```python
from build123d import *

# Parameters (mm, degrees)
SKETCH1_W           = 500
SKETCH1_H           = 150
SKETCH1_R           = 9.3
SKETCH1_R_2         = 3
SKETCH1_R_3         = 4
BOSS_EXTRUDE1_DEPTH = 6.35
CUT_EXTRUDE1_DEPTH  = 7
SKETCH4_R           = 9.3
CUT_EXTRUDE2_DEPTH  = 10
FILLET1_R           = 2
CUT_EXTRUDE4_DEPTH  = 10
SKETCH6_R           = 1.75
SKETCH6_R_2         = 3
CUT_EXTRUDE5_DEPTH  = 10


with BuildPart() as part:
    # Sketch1 → Boss-Extrude1 (new body)
    with BuildSketch(Plane.XY):
        with Locations((200, 0)):
            Rectangle(SKETCH1_W, SKETCH1_H)
        Circle(SKETCH1_R, mode=Mode.SUBTRACT)
        with BuildLine():
            ThreePointArc((303.793920425, 21.250000148), (340.59999997, 42.5), (377.406079545, 21.250000201))
            ThreePointArc((377.406079545, 21.250000201), (375.758965412, 15.102885723), (369.61185099, 16.750000063))
            ThreePointArc((369.61185099, 16.750000063), (340.600001147, 33.5), (311.588150157, 16.750002051))
            ThreePointArc((311.588150157, 16.750002051), (305.441035607, 15.102885134), (303.793920425, 21.250000148))
        make_face(mode=Mode.SUBTRACT)
        with Locations((377.1687, -9.7841)):
            Circle(SKETCH1_R_2, mode=Mode.SUBTRACT)
        with Locations((340.6, 0)):
            Circle(SKETCH1_R_3, mode=Mode.SUBTRACT)
    extrude(amount=BOSS_EXTRUDE1_DEPTH)

    # Sketch3 → Cut-Extrude1 (cut)
    with BuildSketch(Plane.XY.offset(6.35)):
        with BuildLine():
            Line((36.827355724, 55), (-50, 55))
            Line((-50, 55), (-50, -75))
            Line((-50, -75), (450, -75))
            Line((450, -75), (450, 55))
            Line((450, 55), (340.6, 55))
            ThreePointArc((340.6, 55), (379.490872965, 38.890872965), (395.6, 0))
            ThreePointArc((395.6, 0), (394.766919757, -9.536498518), (392.292916219, -18.7841))
            ThreePointArc((392.292916219, -18.7841), (329.589221669, -53.886573101), (285.681879129, 3))
            Line((285.681879129, 3), (30.896152423, 3))
            Line((30.896152423, 3), (21.172644276, 3))
            Line((21.172644276, 3), (9.086322138, -9.086322138))
            ThreePointArc((9.086322138, -9.086322138), (-9.086322138, -9.086322138), (-9.086322138, 9.086322138))
            Line((-9.086322138, 9.086322138), (36.827355724, 55))
        make_face()
        with BuildLine():
            Line((328.4653389, 3), (285.681879129, 3))
            ThreePointArc((285.681879129, 3), (329.589221669, -53.886573101), (392.292916219, -18.7841))
            Line((392.292916219, -18.7841), (371.532319214, -18.7841))
            Line((371.532319214, -18.7841), (351.002913897, -6.930323401))
            ThreePointArc((351.002913897, -6.930323401), (335.559903988, -11.438856245), (328.4653389, 3))
        make_face()
        Polygon((-50, 75), (-50, 55), (36.827355724, 55), (340.6, 55), (450, 55), (450, 75), align=None)
    extrude(amount=-CUT_EXTRUDE1_DEPTH, mode=Mode.SUBTRACT)

    # Sketch4 → Cut-Extrude2 (cut)
    with BuildSketch(Plane.XY.offset(6.35)):
        with BuildLine():
            Line((23.112698372, 8), (6.470027048, 24.642671324))
            Line((6.470027048, 24.642671324), (-9.086322138, 9.086322138))
            ThreePointArc((-9.086322138, 9.086322138), (4.917482106, 11.871851993), (12.85, 0))
            ThreePointArc((12.85, 0), (11.871851993, -4.917482106), (9.086322138, -9.086322138))
            Line((9.086322138, -9.086322138), (21.172644276, 3))
            Line((21.172644276, 3), (41, 3))
            Line((41, 3), (41, 8))
            Line((41, 8), (23.112698372, 8))
        make_face()
        with BuildLine():
            ThreePointArc((12.85, 0), (4.917482106, 11.871851993), (-9.086322138, 9.086322138))
            ThreePointArc((-9.086322138, 9.086322138), (-9.086322138, -9.086322138), (9.086322138, -9.086322138))
            ThreePointArc((9.086322138, -9.086322138), (11.871851993, -4.917482106), (12.85, 0))
        make_face()
        Circle(SKETCH4_R, mode=Mode.SUBTRACT)
        Polygon((36.827355724, 55), (30.827355724, 49), (50.827355724, 49), (50.827355724, 55), align=None)
    extrude(amount=-CUT_EXTRUDE2_DEPTH, mode=Mode.SUBTRACT)

    # Fillet1
    fillet1_edges = [part.edges().sort_by_distance(p)[0] for p in [
        (328.4653389, 3, 3.175),
        (351.002913897, -6.930323401, 3.175),
        (392.292916219, -18.7841, 3.175),
    ]]
    fillet(fillet1_edges, radius=FILLET1_R)

    # Sketch5 → Cut-Extrude4 (cut)
    with BuildSketch(Plane.XY.offset(6.35)):
        with BuildLine():
            ThreePointArc((328.129761947, 0.862068966), (332.07139701, 9.138540969), (340.6, 12.5))
            Line((340.6, 12.5), (394.160713214, 12.5))
            ThreePointArc((394.160713214, 12.5), (374.786985828, 43.084219849), (340.6, 55))
            Line((340.6, 55), (50.827355724, 55))
            Line((50.827355724, 55), (50.827355724, 49))
            Line((50.827355724, 49), (30.827355724, 49))
            Line((30.827355724, 49), (6.470027048, 24.642671324))
            Line((6.470027048, 24.642671324), (23.112698372, 8))
            Line((23.112698372, 8), (41, 8))
            Line((41, 8), (41, 3))
            Line((41, 3), (326.134523859, 3))
            ThreePointArc((326.134523859, 3), (327.596690413, 2.364576478), (328.129761947, 0.862068966))
        make_face()
        with BuildLine():
            ThreePointArc((311.588150157, 16.750002051), (305.441035607, 15.102885134), (303.793920425, 21.250000148))
            ThreePointArc((303.793920425, 21.250000148), (340.59999997, 42.5), (377.406079545, 21.250000201))
            ThreePointArc((377.406079545, 21.250000201), (375.758965412, 15.102885723), (369.61185099, 16.750000063))
            ThreePointArc((369.61185099, 16.750000063), (340.600001147, 33.5), (311.588150157, 16.750002051))
        make_face(mode=Mode.SUBTRACT)
    extrude(amount=-CUT_EXTRUDE4_DEPTH, mode=Mode.SUBTRACT)


with BuildPart() as cut_extrude4_kept_piece:
    # of the separate pieces the step leaves, the one the design keeps (cut_extrude4_pieces_kept)
    add(part.part.solids().sort_by_distance((340.6, 12.5, 0))[0])

    # Sketch6 → Cut-Extrude5 (cut)
    with BuildSketch(Plane.XY.offset(6.35)):
        with Locations((350.6, 7.5)):
            Circle(SKETCH6_R)
        with Locations((387.1687, 0)):
            Circle(SKETCH6_R)
        with Locations((377.1687, -9.7841)):
            Circle(SKETCH6_R_2)
        with Locations((365.870678247, -10.944141097)):
            Circle(SKETCH6_R)
    extrude(amount=-CUT_EXTRUDE5_DEPTH, mode=Mode.SUBTRACT)


solid = cut_extrude4_kept_piece.part
```
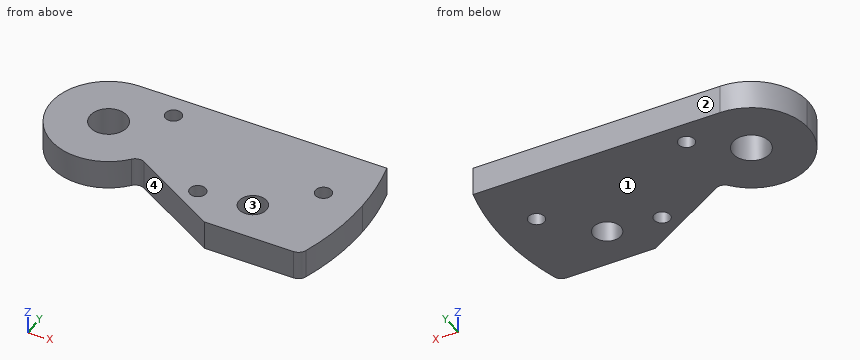
For this review, take the finished solid that the model builds, in its own axes (mm). Face numbers are marked on the shaded views. Round coordinates to 2 decimals unless told otherwise and drop trailing zeros. Order: outer loops, then holes, each group sorted by start corner. A loop starts at its lowest first (then second) coordinate and runs counter-clockwise, first axis right, second up.
Q1. We need section D-D, the plane x = 363. Give the boundary of the cut face in (y, z), plus the area to 3 significant figures.
Findings below:
outline: (-13.86, 0) - (12.5, 0) - (12.5, 6.35) - (-13.86, 6.35) - close
area: 167 mm2
Q2. Mouldability with a two-part tool opening along Y and no side actions: class the marked faces 1, 2, 3 and 4 as pulls with the +Y half, pulls with the -Y half, needs draft (parallel to the pull), parting line crosses it, or undercut.
Findings below:
face 1: needs draft
face 2: pulls with the +Y half
face 3: undercut
face 4: pulls with the -Y half
Q3. We need section C-C, the plane x = 338.5. Give the boundary of the cut face in (y, z), plus the area to 3 significant figures.
Findings below:
outline: (-12.32, 0) - (-3.4, 0) - (-3.4, 6.35) - (-12.32, 6.35) - close; (3.4, 0) - (12.32, 0) - (12.32, 6.35) - (3.4, 6.35) - close
area: 113 mm2
Q4. Insertion check: P1, Ø12, axis at x = 354, y = 7, coming from the -Z side; P2, Ø1, axis at y = 9, z = 2, coming from the -X side; P3, Ø2, axis at x = 368, z = 0.5, coming from the -Y side. Each pin has a flat end and moves straight along its axis. Give the tip position at first contact, or say it passes through.
Findings below:
P1: stops at z = 0
P2: stops at x = 331.43
P3: stops at y = -17.32
Q5. We need section B-B, the plane z = 4. Give the boundary of the cut face in (x, y).
Findings below:
outline: (340.6, 12.5) arc R12.5 ccw (long way) to (350.01, -8.22) arc R2 cw to (352.52, -7.81) - (371.53, -18.78) - (390.87, -18.78) arc R2 ccw to (392.77, -17.42) arc R55 ccw to (394.16, 12.5) - close; hole circle Ø8 at (340.6, 0); hole circle Ø3.5 at (350.6, 7.5); hole circle Ø3.5 at (365.87, -10.94); hole circle Ø6 at (377.17, -9.78); hole circle Ø3.5 at (387.17, 0)
Q6. Wall thickness on line 1 (Y direction, x = 350.5, z = 1.25); line 2 (Y direction, x = 340.6, z = 2.5); line 3 (X direction, y = 1, z = 2.75): over which ranges is each line inside the solid? List them lowest first.
Findings below:
line 1: y = -7.82 to 5.75, 9.25 to 12.5
line 2: y = -12.5 to -4, 4 to 12.5
line 3: x = 328.14 to 336.73, 344.47 to 385.73, 388.6 to 395.59
Q7. We need section A-A, the plane y = -2.5. Give the boundary of the cut face in (x, z).
Findings below:
outline: (328.35, 0) - (337.48, 0) - (337.48, 6.35) - (328.35, 6.35) - close; (343.72, 0) - (395.54, 0) - (395.54, 6.35) - (343.72, 6.35) - close
